Verification items for the finished model (mm, model axes). A direction names the side the tool comes from. Coordinates: 2 decimals unless noted, no trailing zeros. Order: outer loops, then holes, each group sorted by start corner. A loop starts at its lowest first (then second) coordinate and runs counter-clockwise, first axis right, second up.
Q1. Cross-section at B-B, the plane x = -80. Record the boundary of the cut face in (y, z), and give its area (3 significant figures).
Q2. Cross-section at D-D, the plane y = 13.5. Record the boundary of the cut face in (x, z).
Q3. Cross-section at C-C, the plane z = -1.5. Record the boundary of the cut face in (x, y).
Q4. Thickness scan on line 1 (X direction, y = -11.5, z = -3); line 2 (Y direction, x = 0.5, z = 0.5); line 3 (Z direction, x = -42, y = 6.5). Record the ranges inside material, lowest first.
Q5. Cross-section at A-A, the plane y = -4. Record the boundary of the cut face in (x, z), and give its area (3 significant figures).
Q6. Depth check by flat-ended pin: P1, Ø12, axis at x = -26, y = 0.5, coming from the -Z side; P2, Ø8, axis at x = -70, z = 11, coming from the -Y side; P3, Ø12, axis at x = -15, y = 7, coming from the -Z side. Enter the tip coordinate at first touch or a pass-through.
Q7. Set-up check for faces 1 (the flat face through (10, 0, 0)), 2 (the cylindrical face through (-42.89, -2.17, -9.76)): record each of +Z, -Z, +X, -X, +Y, -Y from which the full face is reachable in a straight line by a thin tool's end or side.
from build123d import *

# Parameters (mm, degrees)
F0_R      = 10
F1_DEPTH  = 87
F1_FACE_R = 10
F2_DEPTH  = 10


with BuildPart() as f1:
    # F0 (on Right) → F1 (new body)
    with BuildSketch(Plane.YZ):
        Circle(F0_R)
    extrude(amount=-F1_DEPTH)

    # F0 (on Right) + F1_face (on face) → F2 (join)
    with BuildSketch(Plane.YZ):
        with BuildLine():
            ThreePointArc((14.9995050606, -0.1218521055), (14.9998762647, -0.0609265554), (15, 0))
            ThreePointArc((15, 0), (13.0207371521, 7.4471742302), (7.6052794647, 12.9290264237))
            ThreePointArc((7.6052794647, 12.9290264237), (0.1218517845, 14.9995050633), (-7.3942259846, 13.0508782114))
            ThreePointArc((-7.3942259846, 13.0508782114), (-12.929026562, 7.6052792295), (-14.9995050623, 0.1218519076))
            ThreePointArc((-14.9995050623, 0.1218519076), (-13.0508782952, -7.3942258367), (-7.6052790755, -12.9290266526))
            ThreePointArc((-7.6052790755, -12.9290266526), (-0.1218515337, -14.9995050653), (7.3942260283, -13.0508781867))
            ThreePointArc((7.3942260283, -13.0508781867), (12.9290265245, -7.6052792932), (14.9995050606, -0.1218521055))
        make_face()
        Circle(F0_R, mode=Mode.SUBTRACT)
        with BuildLine():
            ThreePointArc((7.6052794647, 12.9290264237), (13.0207371521, 7.4471742302), (15, 0))
            ThreePointArc((15, 0), (14.9998762647, -0.0609265554), (14.9995050606, -0.1218521055))
            Line((14.9995050606, -0.1218521055), (15.0698562292, 8.5381164921))
            Line((15.0698562292, 8.5381164921), (7.6052794647, 12.9290264237))
        make_face()
        with BuildLine():
            ThreePointArc((-7.3942259846, 13.0508782114), (0.1218517845, 14.9995050633), (7.6052794647, 12.9290264237))
            Line((7.6052794647, 12.9290264237), (0.140702332, 17.3199365719))
            Line((0.140702332, 17.3199365719), (-7.3942259846, 13.0508782114))
        make_face()
        with BuildLine():
            Line((14.9291538972, -8.7818200798), (14.9995050606, -0.1218521055))
            ThreePointArc((14.9995050606, -0.1218521055), (12.9290265245, -7.6052792932), (7.3942260283, -13.0508781867))
            Line((7.3942260283, -13.0508781867), (14.9291538972, -8.7818200798))
        make_face()
        with BuildLine():
            ThreePointArc((-14.9995050623, 0.1218519076), (-12.929026562, 7.6052792295), (-7.3942259846, 13.0508782114))
            Line((-7.3942259846, 13.0508782114), (-14.9291538972, 8.7818200798))
            Line((-14.9291538972, 8.7818200798), (-14.9995050623, 0.1218519076))
        make_face()
        with BuildLine():
            Line((-0.140702332, -17.3199365719), (7.3942260283, -13.0508781867))
            ThreePointArc((7.3942260283, -13.0508781867), (-0.1218515337, -14.9995050653), (-7.6052790755, -12.9290266526))
            Line((-7.6052790755, -12.9290266526), (-0.140702332, -17.3199365719))
        make_face()
        with BuildLine():
            ThreePointArc((-7.6052790755, -12.9290266526), (-13.0508782952, -7.3942258367), (-14.9995050623, 0.1218519076))
            Line((-14.9995050623, 0.1218519076), (-15.0698562292, -8.5381164921))
            Line((-15.0698562292, -8.5381164921), (-7.6052790755, -12.9290266526))
        make_face()
    with BuildSketch(Plane.YZ):
        Circle(F1_FACE_R)
    extrude(amount=F2_DEPTH)


solid = f1.part
Check values:
1. outline: circle Ø20 at (0, 0)
1. area: 314 mm2
2. outline: (0, -9.59) - (10, -9.59) - (10, 9.46) - (0, 9.46) - close
3. outline: (-87, -9.89) - (0, -9.89) - (0, -15.01) - (10, -15.01) - (10, 14.99) - (0, 14.99) - (0, 9.89) - (-87, 9.89) - close
4. line 1: x = 0 to 10
4. line 2: y = -15 to 15
4. line 3: z = -7.6 to 7.6
5. outline: (-87, -9.17) - (0, -9.17) - (0, -15.05) - (10, -15.05) - (10, 14.97) - (0, 14.97) - (0, 9.17) - (-87, 9.17) - close
5. area: 1,890 mm2
6. P1: stops at z = -10
6. P2: stops at y = -7.14
6. P3: stops at z = -9.95
7. face 1: +Z, -Z, +X, +Y, -Y
7. face 2: -X
